Design review of the part built by this model. Coordinates are the model's own, in mm. Face numbers are marked on the shaded views. A direction names the side the tool comes from. Give positions to 0.01 mm unless a question says otherwise; leave off trailing zeros. Write each loop counter-clockwise with the first axis right and the second up, starting at its lowest first coordinate (ties: lowest second). Pieces come first, ordered by that corner, then holes. Notation, with made-up numbers: (71, 15) -> (88, 15) arc R23 cw to (88, 53) -> close; hole circle Ø8 at (-32.75, 6). An arc over 180 degrees is marked (long way). Put each result on its own line as item: value. Start each with the question number.
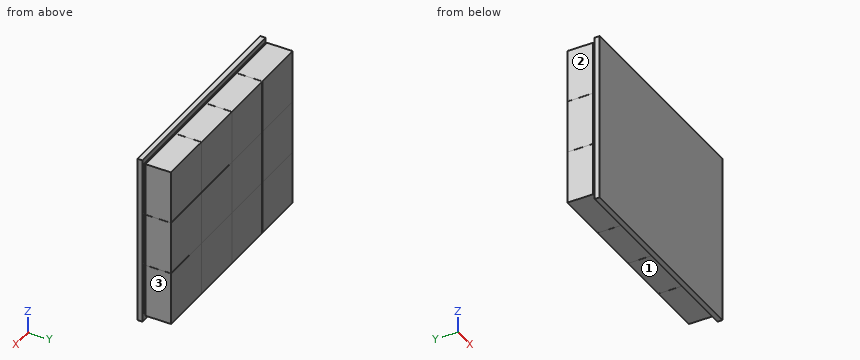
from build123d import *

# Parameters (mm, degrees)
SKETCH1_W                  = 500
SKETCH1_H                  = 166
BOSS_EXTRUDE1_DEPTH        = 5
SKETCH2_W                  = 50
SKETCH2_H                  = 50
BOSS_EXTRUDE3_DEPTH        = 2
LPATTERN1_COUNT            = 3
LPATTERN1_PITCH            = 52
SKETCH3_W                  = 52
SKETCH3_H                  = 51.9
BOSS_EXTRUDE8_DEPTH        = 25
LPATTERN5_COUNT            = 3
LPATTERN5_PITCH            = 52
LPATTERN6_COUNT            = 4
LPATTERN6_PITCH            = 52.1
LPATTERN6_COPY_1_SKETCH_W  = 50
LPATTERN6_COPY_1_SKETCH_H  = 50
LPATTERN6_COPY_1_DEPTH     = 2
LPATTERN6_COPY_2_SKETCH_W  = 50
LPATTERN6_COPY_2_SKETCH_H  = 50
LPATTERN6_COPY_2_DEPTH     = 2
LPATTERN6_COPY_3_SKETCH_W  = 50
LPATTERN6_COPY_3_SKETCH_H  = 50
LPATTERN6_COPY_3_DEPTH     = 2
LPATTERN6_COPY_4_SKETCH_W  = 50
LPATTERN6_COPY_4_SKETCH_H  = 50
LPATTERN6_COPY_4_DEPTH     = 2
LPATTERN6_COPY_5_SKETCH_W  = 50
LPATTERN6_COPY_5_SKETCH_H  = 50
LPATTERN6_COPY_5_DEPTH     = 2
LPATTERN6_COPY_6_SKETCH_W  = 50
LPATTERN6_COPY_6_SKETCH_H  = 50
LPATTERN6_COPY_6_DEPTH     = 2
LPATTERN6_COPY_7_SKETCH_W  = 52
LPATTERN6_COPY_7_SKETCH_H  = 51.9
LPATTERN6_COPY_7_DEPTH     = 25
LPATTERN6_COPY_8_SKETCH_W  = 52
LPATTERN6_COPY_8_SKETCH_H  = 51.9
LPATTERN6_COPY_8_DEPTH     = 25
LPATTERN6_COPY_9_SKETCH_W  = 52
LPATTERN6_COPY_9_SKETCH_H  = 51.9
LPATTERN6_COPY_9_DEPTH     = 25
LPATTERN6_COPY_10_SKETCH_W = 52
LPATTERN6_COPY_10_SKETCH_H = 51.9
LPATTERN6_COPY_10_DEPTH    = 25
LPATTERN6_COPY_11_SKETCH_W = 52
LPATTERN6_COPY_11_SKETCH_H = 51.9
LPATTERN6_COPY_11_DEPTH    = 25
LPATTERN6_COPY_12_SKETCH_W = 52
LPATTERN6_COPY_12_SKETCH_H = 51.9
LPATTERN6_COPY_12_DEPTH    = 25
SKETCH4_W                  = 223.089941366
SKETCH4_H                  = 166
SKETCH4_W_2                = 66.355147464
CUT_EXTRUDE1_DEPTH         = 10


with BuildPart() as part:
    # Sketch1 → Boss-Extrude1 (new body)
    with BuildSketch(Plane(origin=(0, 0, 0), x_dir=(1, 0, 0), z_dir=(0, 1, 0))):
        Rectangle(SKETCH1_W, SKETCH1_H)
    extrude(amount=BOSS_EXTRUDE1_DEPTH)

    # Sketch2 → Boss-Extrude3 (add)
    with BuildSketch(Plane(origin=(0, 5, 0), x_dir=(1, 0, 0), z_dir=(0, 1, 0))):
        with Locations((0, -53)):
            Rectangle(SKETCH2_W, SKETCH2_H)
    boss_extrude3 = extrude(amount=BOSS_EXTRUDE3_DEPTH)

    # LPattern1: Boss-Extrude3 ×3
    with Locations(*[(0, 0, -i * LPATTERN1_PITCH) for i in range(1, LPATTERN1_COUNT)]):
        add(boss_extrude3)

    # Sketch3 → Boss-Extrude8 (add)
    with BuildSketch(Plane(origin=(0, 7, 0), x_dir=(1, 0, 0), z_dir=(0, 1, 0))):
        with Locations((0, -53.05)):
            Rectangle(SKETCH3_W, SKETCH3_H)
    boss_extrude8 = extrude(amount=BOSS_EXTRUDE8_DEPTH)

    # LPattern5: Boss-Extrude8 ×3
    with Locations(*[(0, 0, -i * LPATTERN5_PITCH) for i in range(1, LPATTERN5_COUNT)]):
        add(boss_extrude8)

    # LPattern6: Boss-Extrude3, Boss-Extrude8 ×4
    with Locations(*[(i * LPATTERN6_PITCH, 0, 0) for i in range(1, LPATTERN6_COUNT)]):
        add(boss_extrude3)
        add(boss_extrude8)

    # LPattern6 copy 1 sketch → LPattern6 copy 1 (add)
    with BuildSketch(Plane(origin=(52.1, 5, -52), x_dir=(1, 0, 0), z_dir=(0, 1, 0))):
        with Locations((0, -53)):
            Rectangle(LPATTERN6_COPY_1_SKETCH_W, LPATTERN6_COPY_1_SKETCH_H)
    extrude(amount=LPATTERN6_COPY_1_DEPTH)

    # LPattern6 copy 2 sketch → LPattern6 copy 2 (add)
    with BuildSketch(Plane(origin=(104.2, 5, -52), x_dir=(1, 0, 0), z_dir=(0, 1, 0))):
        with Locations((0, -53)):
            Rectangle(LPATTERN6_COPY_2_SKETCH_W, LPATTERN6_COPY_2_SKETCH_H)
    extrude(amount=LPATTERN6_COPY_2_DEPTH)

    # LPattern6 copy 3 sketch → LPattern6 copy 3 (add)
    with BuildSketch(Plane(origin=(156.3, 5, -52), x_dir=(1, 0, 0), z_dir=(0, 1, 0))):
        with Locations((0, -53)):
            Rectangle(LPATTERN6_COPY_3_SKETCH_W, LPATTERN6_COPY_3_SKETCH_H)
    extrude(amount=LPATTERN6_COPY_3_DEPTH)

    # LPattern6 copy 4 sketch → LPattern6 copy 4 (add)
    with BuildSketch(Plane(origin=(52.1, 5, -104), x_dir=(1, 0, 0), z_dir=(0, 1, 0))):
        with Locations((0, -53)):
            Rectangle(LPATTERN6_COPY_4_SKETCH_W, LPATTERN6_COPY_4_SKETCH_H)
    extrude(amount=LPATTERN6_COPY_4_DEPTH)

    # LPattern6 copy 5 sketch → LPattern6 copy 5 (add)
    with BuildSketch(Plane(origin=(104.2, 5, -104), x_dir=(1, 0, 0), z_dir=(0, 1, 0))):
        with Locations((0, -53)):
            Rectangle(LPATTERN6_COPY_5_SKETCH_W, LPATTERN6_COPY_5_SKETCH_H)
    extrude(amount=LPATTERN6_COPY_5_DEPTH)

    # LPattern6 copy 6 sketch → LPattern6 copy 6 (add)
    with BuildSketch(Plane(origin=(156.3, 5, -104), x_dir=(1, 0, 0), z_dir=(0, 1, 0))):
        with Locations((0, -53)):
            Rectangle(LPATTERN6_COPY_6_SKETCH_W, LPATTERN6_COPY_6_SKETCH_H)
    extrude(amount=LPATTERN6_COPY_6_DEPTH)

    # LPattern6 copy 7 sketch → LPattern6 copy 7 (add)
    with BuildSketch(Plane(origin=(52.1, 7, -52), x_dir=(1, 0, 0), z_dir=(0, 1, 0))):
        with Locations((0, -53.05)):
            Rectangle(LPATTERN6_COPY_7_SKETCH_W, LPATTERN6_COPY_7_SKETCH_H)
    extrude(amount=LPATTERN6_COPY_7_DEPTH)

    # LPattern6 copy 8 sketch → LPattern6 copy 8 (add)
    with BuildSketch(Plane(origin=(104.2, 7, -52), x_dir=(1, 0, 0), z_dir=(0, 1, 0))):
        with Locations((0, -53.05)):
            Rectangle(LPATTERN6_COPY_8_SKETCH_W, LPATTERN6_COPY_8_SKETCH_H)
    extrude(amount=LPATTERN6_COPY_8_DEPTH)

    # LPattern6 copy 9 sketch → LPattern6 copy 9 (add)
    with BuildSketch(Plane(origin=(156.3, 7, -52), x_dir=(1, 0, 0), z_dir=(0, 1, 0))):
        with Locations((0, -53.05)):
            Rectangle(LPATTERN6_COPY_9_SKETCH_W, LPATTERN6_COPY_9_SKETCH_H)
    extrude(amount=LPATTERN6_COPY_9_DEPTH)

    # LPattern6 copy 10 sketch → LPattern6 copy 10 (add)
    with BuildSketch(Plane(origin=(52.1, 7, -104), x_dir=(1, 0, 0), z_dir=(0, 1, 0))):
        with Locations((0, -53.05)):
            Rectangle(LPATTERN6_COPY_10_SKETCH_W, LPATTERN6_COPY_10_SKETCH_H)
    extrude(amount=LPATTERN6_COPY_10_DEPTH)

    # LPattern6 copy 11 sketch → LPattern6 copy 11 (add)
    with BuildSketch(Plane(origin=(104.2, 7, -104), x_dir=(1, 0, 0), z_dir=(0, 1, 0))):
        with Locations((0, -53.05)):
            Rectangle(LPATTERN6_COPY_11_SKETCH_W, LPATTERN6_COPY_11_SKETCH_H)
    extrude(amount=LPATTERN6_COPY_11_DEPTH)

    # LPattern6 copy 12 sketch → LPattern6 copy 12 (add)
    with BuildSketch(Plane(origin=(156.3, 7, -104), x_dir=(1, 0, 0), z_dir=(0, 1, 0))):
        with Locations((0, -53.05)):
            Rectangle(LPATTERN6_COPY_12_SKETCH_W, LPATTERN6_COPY_12_SKETCH_H)
    extrude(amount=LPATTERN6_COPY_12_DEPTH)

    # Sketch4 → Cut-Extrude1 (cut)
    with BuildSketch(Plane(origin=(0, 5, 0), x_dir=(1, 0, 0), z_dir=(0, 1, 0))):
        with Locations((-138.455029317, 0)):
            Rectangle(SKETCH4_W, SKETCH4_H)
        with Locations((216.822426268, 0)):
            Rectangle(SKETCH4_W_2, SKETCH4_H)
    extrude(amount=-CUT_EXTRUDE1_DEPTH, mode=Mode.SUBTRACT)


solid = part.part
Q1. Take a section at A-A on x = -6.5. Give the boundary of the cut face in (y, z).
Q2. For pin 1 (12.5 mm diameter, centred on x = 107, y = 15, fed in from -Z); pin 2 (7.5 mm diameter, centred on x = 44.5, y = 13.5, fed in from +Z); pin 3 (12 mm diameter, centred on y = 15, z = -11, fed in from -X), all flat-tipped, find the tip position at first contact; note any pin that passes through.
Q3. Take a section at B-B on y = 28.5. State how many separate pieces and enclosed holes the cut face has, then the cut area to 3 significant figures.
Q4. To check wall thickness, follow probe 1 along X at (y, z) = (6, 30). State the ranges of the line that lie inside material, in increasing order. Write a range as from..to.
Q5. Machinability: for the marked faces 1, 2 and 3, which of the approach directions +Z, -Z, +X, -X, +Y, -Y give a long, thin tool a straight path to every point of the face, cutting with its end or side? Answer none if there is none.
Result:
1. outline: (0, -83) -> (5, -83) -> (5, -76) -> (7, -76) -> (7, -76.9) -> (32, -76.9) -> (32, -25) -> (7, -25) -> (7, -26) -> (5, -26) -> (5, -24) -> (7, -24) -> (7, -24.9) -> (32, -24.9) -> (32, 27) -> (7, 27) -> (7, 26) -> (5, 26) -> (5, 28) -> (7, 28) -> (7, 27.1) -> (32, 27.1) -> (32, 79) -> (7, 79) -> (7, 78) -> (5, 78) -> (5, 83) -> (0, 83) -> close
2. pin 1: stops at z = -76.9
2. pin 2: stops at z = 79
2. pin 3: stops at x = -26
3. separate pieces: 12
3. enclosed holes: 0
3. area: 32,400 mm^2
4. probe 1: x = -25..25, 27.1..77.1, 79.2..129.2, 131.3..181.3
5. face 1: -Z, +X, -X, +Y
5. face 2: +Z, -Z, -X, +Y
5. face 3: +Z, -Z, +X, +Y
